The model under review builds one solid part; all positions refer to its coordinate system, in mm. A direction names the side the tool comes from. Round coordinates to 2 decimals unless told otherwise and drop trailing zeros. Write each loop counter-clockwise with the first axis right and the second up, starting at its lowest first coordinate (ties: lowest second). Pieces come first, ordered by that corner, then holes.
Item 1: Add section B-B (x = -61). Give the boundary of the cut face in (y, z) (3 decimals).
Item 2: Machinability: for faces 3 (the face through (1, 2, 2.5)), 4 (the face through (-63, 2, -2)), 5 (the face through (-1, 2, -2.5)), which of the approach directions +Z, -Z, +X, -X, +Y, -Y give a long, thin tool a straight path to every point of the face, cutting with its end or side? Answer none if there is none.
Item 3: Add section D-D (x = 1). Give the boundary of the cut face in (y, z).
Item 4: Add section C-C (y = 1.05). Give the boundary of the cut face in (x, z) (3 decimals).
Item 5: Add section A-A (z = 0). Give the boundary of the cut face in (x, y) (3 decimals).
Item 6: Draft analysis for pull direction X (two halves, no side actions). For faces 1 (the face through (-1, 0, 0)), 2 (the face through (57.55, 2.03, -0.4)), state which applies: +X half, -X half, draft (parallel to the pull), parting line (faces both ways), or undercut.
Item 7: Clearance check with flat-ended pins moving along their axes: pin 1 Ø2 at (x, y) = (-10.5, 1) entering from -Z; pin 2 Ø2 at (x, z) = (-61.5, 1.5) entering from -Y; pin 3 Ø1 at (y, z) = (2.5, 3) entering from -X. State where each tip first meets the part, or that it passes through.
Item 8: To check wall thickness, follow L1, parallel to Z at x = 17, y = 2.6; L2, parallel to X at y = 3.4, z = 4.25; L3, parallel to X at y = 2.85, z = -2. State the ranges of each line that lie inside material, in increasing order.
```python
from build123d import *

# Parameters (mm, degrees)
BOSS_EXTRUDE1_DEPTH = 4
SKETCH3_R           = 3.5
CUT_EXTRUDE2_DEPTH  = 2
SKETCH2_R           = 1.825
CUT_EXTRUDE1_DEPTH  = 68.930111144


with BuildPart() as part:
    # Sketch1 → Boss-Extrude1 (new body)
    with BuildSketch(Plane(origin=(0, 0, 0), x_dir=(1, 0, 0), z_dir=(0, 1, 0))):
        with BuildLine():
            Line((-55, 2.5), (55, 2.5))
            ThreePointArc((55, 2.5), (64.330127019, 0), (55, -2.5))
            Line((55, -2.5), (-55, -2.5))
            ThreePointArc((-55, -2.5), (-67.5, 0), (-55, 2.5))
        make_face()
    extrude(amount=BOSS_EXTRUDE1_DEPTH)

    # Sketch3 → Cut-Extrude2 (cut)
    with BuildSketch(Plane.XZ):
        with Locations(Location((-61, 0, 0), (0, 0, 270))):
            Circle(SKETCH3_R)
    extrude(amount=-CUT_EXTRUDE2_DEPTH, mode=Mode.SUBTRACT)

    # Sketch2 → Cut-Extrude1 (cut, through all)
    with BuildSketch(Plane(origin=(0, 4, 0), x_dir=(1, 0, 0), z_dir=(0, 1, 0))):
        with Locations(Location((-61, 0, 0), (0, 0, 270))):
            Circle(SKETCH2_R)
        with Locations(Location((59.330127019, 0, 0), (0, 0, 270))):
            Circle(SKETCH2_R)
    extrude(amount=-CUT_EXTRUDE1_DEPTH, mode=Mode.SUBTRACT)


solid = part.part
```
Numbers:
1. outline: (0, -6.5) - (4, -6.5) - (4, -1.825) - (2, -1.825) - (2, -3.5) - (0, -3.5) - close; (0, 3.5) - (2, 3.5) - (2, 1.825) - (4, 1.825) - (4, 6.5) - (0, 6.5) - close
2. face 3: +Z, +Y, -Y
2. face 4: -Y
2. face 5: -Z, +Y, -Y
3. outline: (0, -2.5) - (4, -2.5) - (4, 2.5) - (0, 2.5) - close
4. outline: (-55, -2.5) - (55, -2.5) arc R5 ccw (long way) to (55, 2.5) - (-55, 2.5) arc R6.5 ccw (long way) to start; hole circle Ø7 at (-61, 0); hole circle Ø3.65 at (59.33, 0)
5. outline: (-67.5, 0) - (-64.5, 0) - (-64.5, 2) - (-62.825, 2) - (-62.825, 4) - (-67.5, 4) - close; (-59.175, 2) - (-57.5, 2) - (-57.5, 0) - (57.505, 0) - (57.505, 4) - (-59.175, 4) - close; (61.155, 0) - (64.33, 0) - (64.33, 4) - (61.155, 4) - close
6. face 1: draft
6. face 2: undercut
7. pin 1: stops at z = -2.5
7. pin 2: stops at y = 2
7. pin 3: stops at x = -67
8. L1: z = -2.5 to 2.5
8. L2: x = -65.92 to -56.08, 56.7 to 61.96
8. L3: x = -67.18 to 63.91
